Design review of the part built by this model. Coordinates are the model's own, in mm. Face numbers are marked on the shaded views. A direction names the side the tool comes from. Coordinates: 2 decimals unless noted, no trailing zeros. Write each loop counter-clockwise with the first axis right and the second up, starting at its lowest first coordinate (ties: lowest second). Pieces come first, ordered by that corner, then holes. Notation, with made-up numbers: (-2, 61) - (51, 61) arc R18 cw to (51, 81) - close; hole circle Ø1 at (-36, 36.25). An arc over 180 degrees is marked (long way). One line per item, written item: value.
from build123d import *

# Parameters (mm, degrees)
F1_DEPTH = 200


with BuildPart() as f1:
    # F0 (on Front) → F1 (new body)
    with BuildSketch(Plane.XZ):
        Polygon((-369.296074, 860.103846), (-252.222359, 781.455187), (-248.795434, 803.075274), (-359.538714, 871.651432), (-369.296074, 877.693534), align=None)
        Polygon((86.229337, 578.00982), (102.297463, 567.215454), (176.989675, 817.272305), (159.574956, 827.140868), align=None)
        Polygon((47.703233, 203.298303), (36.957281, 149.250944), (177.764803, 223.871082), (177.764803, 265.354425), align=None)
        Polygon((-395.137998, 184.585006), (-382.793993, 195.368357), (-488.34646, 285.545486), (-488.302618, 285.309941), (-488.635778, 274.76051), align=None)
        Polygon((-531.360984, 110.484615), (-379.167348, 166.403156), (-402.947897, 177.762512), (-531.832361, 122.413635), align=None)
        Polygon((2.565403, -500.237301), (16.359659, -532.357335), (319.279872, -428.741529), (305.078506, -405.49764), align=None)
        Polygon((-19.985075, 296.750159), (-4.052614, 274.753479), (86.380119, 425.346863), (115.178615, 473.303646), (90.32318, 474.886388), align=None)
        Polygon((-27.504601, -522.620559), (16.359659, -532.357335), (2.565403, -500.237301), (-98.492666, -264.92278), (-98.84321, -264.855158), (-131.214753, -258.610427), (-140.553485, -256.808911), (-137.378573, -264.274074), (-127.665923, -287.111413), align=None)
        Polygon((-24.854315, -64.498566), (-44.484516, -96.92555), (450.421533, 36.795169), (467.866212, 41.508619), (451.568961, 61.298091), align=None)
        Polygon((-348.866686, -310.636839), (-273.434583, -255.175081), (-273.434583, -231.175081), (-291.156466, -244.943347), (-348.866686, -289.778855), align=None)
        Polygon((-379.167348, 166.403156), (-32.11826, 0.626743), (-23.780994, 24.570884), (-382.793993, 195.368357), (-395.137998, 184.585006), (-402.947897, 177.762512), align=None)
        Polygon((-439.231479, 462.925151), (-424.822895, 458.121201), (-463.330506, 606.581709), (-472.21759, 605.160534), align=None)
        Polygon((115.178615, 473.303646), (86.380119, 425.346863), (437.898695, 581.404746), (418.918312, 604.574621), align=None)
        Polygon((-404.833034, 721.9197), (-235.007594, 769.890523), (-252.222359, 781.455187), (-407.638371, 730.471313), align=None)
        Polygon((-135.523954, 354.126599), (-119.959313, 346.397221), (-133.090726, 431.585663), (-186.222941, 528.623852), (-193.045956, 522.75474), (-146.845546, 425.733876), align=None)
        Polygon((458.64677, 613.760918), (437.898695, 581.404746), (726.593494, 539.26003), (726.593494, 556.879818), align=None)
        Polygon((636.286535, 776.768744), (522.923824, 744.332003), (536.942677, 735.861683), (639.587648, 765.231731), align=None)
        Polygon((467.866212, 41.508619), (450.421533, 36.795169), (666.4446, 25.382621), (793.553748, -8.556767), (796.343327, 0), (669.01958, 41.508619), (480.751061, 50.054641), align=None)
        Polygon((335.479707, -405.49764), (319.279872, -428.741529), (568.452358, -431.648523), (565.515757, -415.986478), align=None)
        Polygon((-23.780994, 24.570884), (0, 13.257272), (36.957281, 149.250944), (6.303291, 133.006038), align=None)
        Polygon((177.764803, 265.354425), (177.764803, 223.871082), (626.504063, 314.041543), (643.625182, 317.481891), (794.811727, 347.861582), (789.644241, 358.691961), (193.296715, 267.723699), align=None)
        Polygon((-435.548306, 448.704898), (-135.523954, 333.758116), (-135.523954, 354.126599), (-424.822895, 458.121201), align=None)
        Polygon((159.574956, 827.140868), (176.989675, 817.272305), (268.250609, 930.605381), (259.307712, 938.606918), align=None)
        Polygon((-291.156466, -244.943347), (-273.434583, -231.175081), (-348.866686, -164.524183), (-348.866686, -179.095539), align=None)
        Polygon((-114.152497, -161.216129), (-86.680702, -166.629118), (-44.484516, -96.92555), (-24.854315, -64.498566), (-53.700276, -61.355551), align=None)
        Polygon((418.918312, 604.574621), (437.898695, 581.404746), (458.64677, 613.760918), (536.942677, 735.861683), (522.923824, 744.332003), align=None)
        Polygon((-367.221205, -159.679715), (-348.866686, -164.524183), (-379.069601, -54.813134), (-386.85894, -60.159795), align=None)
        Polygon((-135.523954, 333.758116), (-32.865988, 275.321412), (-19.985075, 296.750159), (-119.959313, 346.397221), (-135.523954, 354.126599), align=None)
        Polygon((-98.84321, -264.855158), (-98.492666, -264.92278), (-98.771259, -264.274074), (-86.680702, -166.629118), (-114.152497, -161.216129), (-131.214753, -258.610427), align=None)
        Polygon((-273.434583, -255.175081), (-127.665923, -287.111413), (-137.378573, -264.274074), (-140.553485, -256.808911), (-273.434583, -231.175081), align=None)
        Polygon((736.995518, 166.414723), (618.033409, 159.081429), (625.630806, 146.147769), (737.853944, 152.489179), align=None)
        Polygon((305.078506, -405.49764), (319.279872, -428.741529), (335.479707, -405.49764), (434.80089, -262.989367), (448.050529, -243.978485), (428.385645, -243.978485), align=None)
        Polygon((18.307742, 176.274624), (47.703233, 203.298303), (-4.052614, 274.753479), (-19.985075, 296.750159), (-32.865988, 275.321412), align=None)
        Polygon((375.046786, -162.758924), (428.385645, -243.978485), (448.050529, -243.978485), (382.328452, -153.220721), align=None)
        Polygon((618.033409, 159.081429), (451.568961, 61.298091), (467.866212, 41.508619), (480.751061, 50.054641), (625.630806, 146.147769), align=None)
        Polygon((-567.206264, 920.252979), (-369.296074, 860.103846), (-369.296074, 877.693534), (-567.206264, 929.252979), align=None)
        Polygon((-235.007594, 769.890523), (69.973044, 565.008342), (96.346088, 547.291261), (102.297463, 567.215454), (86.229337, 578.00982), (-248.795434, 803.075274), (-252.222359, 781.455187), align=None)
        Polygon((69.973044, 565.008342), (90.32318, 474.886388), (115.178615, 473.303646), (96.346088, 547.291261), align=None)
        Polygon((-26, -750), (0, -750), (26, -750), (16.359659, -532.357335), (-27.504601, -522.620559), align=None)
        Polygon((177.764803, 342.098653), (177.764803, 265.354425), (193.296715, 267.723699), (189.764803, 342.098653), align=None)
        Polygon((-496.074945, -135.48176), (-496.71203, -125.502074), (-548.627883, -146.178946), (-548.627883, -153.460398), align=None)
        Polygon((726.593494, 556.879818), (726.593494, 539.26003), (771.621823, 491.295099), (778.099352, 501.396665), align=None)
        Polygon((-348.866686, -179.095539), (-348.866686, -164.524183), (-367.221205, -159.679715), (-496.71203, -125.502074), (-496.074945, -135.48176), align=None)
        Polygon((565.515757, -415.986478), (568.452358, -431.648523), (635.317527, -359.778498), (628.163874, -354.317248), align=None)
        Polygon((-369.296074, 877.693534), (-359.538714, 871.651432), (-368.308287, 948.842063), (-375.864416, 943.952799), align=None)
        Polygon((-531.10688, 485.458205), (-435.548306, 448.704898), (-424.822895, 458.121201), (-439.231479, 462.925151), (-528.345922, 492.636694), align=None)
        Polygon((-573.983948, 295.886798), (-488.635778, 274.76051), (-488.302618, 285.309941), (-573.983948, 305.886798), align=None)
        Polygon((6.303291, 133.006038), (36.957281, 149.250944), (47.703233, 203.298303), (18.307742, 176.274624), align=None)
        Polygon((239.989832, 429.213673), (177.764803, 342.098653), (189.764803, 342.098653), (247.313433, 423.982528), align=None)
        Polygon((-386.85894, -60.159795), (-379.069601, -54.813134), (-474.725813, 18.311166), (-474.725813, 11.253227), align=None)
        Polygon((643.625182, 317.481891), (626.504063, 314.041543), (696.974933, 268.784612), (708.739766, 271.148659), align=None)
        Polygon((-32.11826, 0.626743), (-53.700276, -61.355551), (-24.854315, -64.498566), (0, 13.257272), (-23.780994, 24.570884), align=None)
        Polygon((448.050529, -243.978485), (434.80089, -262.989367), (646.405697, -255.978485), (646.405697, -243.978485), align=None)
        Polygon((-551.066445, 122.413635), (-531.360984, 110.484615), (-531.832361, 122.413635), (-568.067963, 144.349445), (-573.983948, 136.287118), align=None)
    extrude(amount=F1_DEPTH)


solid = f1.part
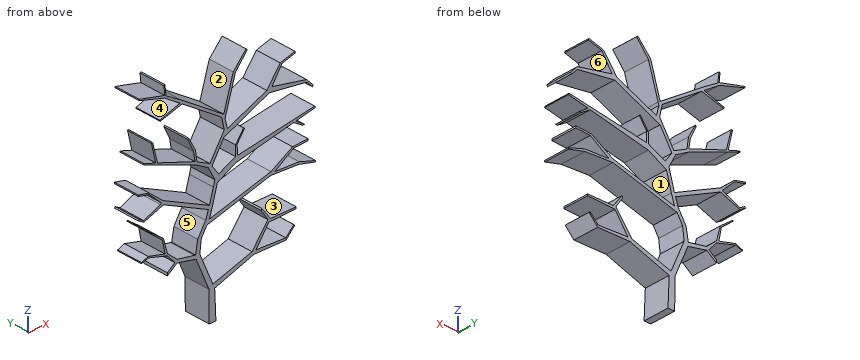
1. Insertion check: pin 1 Ø5 at (y, z) = (-71, 115) entering from -X; pin 2 Ø5 at (x, y) = (204.5, -64) entering from +Z; pin 3 Ø6 at (y, z) = (-111, -248.5) entering from +X. Each pin has a flat end and moves straight along its axis. Give the tip position at first contact, or say it passes through.
Answer block:
pin 1: stops at x = -542.95
pin 2: stops at z = 880.15
pin 3: stops at x = 646.41
2. For the marked faces 1, 2 and 3, list the 3-axis set-ups (+Z, -Z, +X, -X, +Y, -Y) from which the entire face can be reached by the end or side of a thin tool; tool diameter is ignored.
Answer block:
face 1: +Y, -Y
face 2: +Z, +Y, -Y
face 3: +X, +Y, -Y
3. Consider section A-A, the plane x = 212.5. Write out the cut boundary in (y, z).
Answer block:
outline: (-200, -465.27) - (0, -465.27) - (0, -434.49) - (-200, -434.49) - close; (-200, -27.49) - (0, -27.49) - (0, -1.83) - (-200, -1.83) - close; (-200, 230.85) - (0, 230.85) - (0, 270.65) - (-200, 270.65) - close; (-200, 374.45) - (0, 374.45) - (0, 390.73) - (-200, 390.73) - close; (-200, 481.34) - (0, 481.34) - (0, 515.36) - (-200, 515.36) - close; (-200, 861.37) - (0, 861.37) - (0, 886.29) - (-200, 886.29) - close
4. Mouldability with a two-part tool opening along X and no side actions: class the marked faces 4, 5 and 6 as released by +X, released by -X, zero draft, split by the parting line, or undercut.
Answer block:
face 4: released by -X
face 5: undercut
face 6: released by +X
5. Wall thickness on line 1 along Z through (x, y) = (-422.5, -54); line 2 along Z through (x, y) = (-303.5, -175.5); line 3 along X through (y, z) = (-126.5, -227.5): over which ranges is each line inside the solid? List them lowest first.
Answer block:
line 1: z = -157.28 to -145.09, -31.19 to -21.61, 150.48 to 169.37, 210.97 to 229.29, 443.71 to 457.29, 876.27 to 891.55
line 2: z = -277.28 to -254.53, -230.86 to -204.61, 130.26 to 157.64, 398.11 to 414.51, 750.54 to 764.63, 815.9 to 836.95
line 3: x = -306.44 to -277.59, -125.76 to -94.22, 417.56 to 436.12
